from build123d import *

# Parameters (mm, degrees)
BOSS_EXTRUDE3_DEPTH = 9.25
SKETCH5_W           = 4
SKETCH5_H           = 0.86
CUT_EXTRUDE1_DEPTH  = 2
SKETCH6_W           = 3.5
SKETCH6_H           = 0.5
BOSS_EXTRUDE4_DEPTH = 0.5
SKETCH7_W           = 0.72
SKETCH7_H           = 2.3359
CUT_EXTRUDE2_DEPTH  = 2
FILLET1_R           = 0.25
FILLET2_R           = 0.1


with BuildPart() as part:
    # Sketch1 → Boss-Extrude3 (new body, symmetric)
    with BuildSketch(Plane(origin=(0, 0, 0), x_dir=(0, 0, -1), z_dir=(1, 0, 0))):
        Polygon((-0.122813016, -2.026219673), (-0.122813016, 0.173780327), (1.877186984, 0.309680327), (1.877186984, -2.026219673), align=None)
    extrude(amount=BOSS_EXTRUDE3_DEPTH, both=True)

    # Sketch5 → Cut-Extrude1 (cut)
    with BuildSketch(Plane(origin=(0, 0, -1.877186984), x_dir=(-1, 0, 0), z_dir=(0, 0, -1))):
        with Locations((-2.34, -0.120319673)):
            Rectangle(SKETCH5_W, SKETCH5_H)
    extrude(amount=-CUT_EXTRUDE1_DEPTH, mode=Mode.SUBTRACT)

    # Sketch6 → Boss-Extrude4 (add)
    with BuildSketch(Plane.XZ.offset(2.026219673)):
        with Locations((0.34, -0.877186984)):
            Rectangle(SKETCH6_W, SKETCH6_H)
    extrude(amount=BOSS_EXTRUDE4_DEPTH)

    # Sketch7 → Cut-Extrude2 (cut)
    with BuildSketch(Plane(origin=(0, 0, -1.877186984), x_dir=(-1, 0, 0), z_dir=(0, 0, -1))):
        with Locations((8.89, -0.858269673)):
            Rectangle(SKETCH7_W, SKETCH7_H)
    extrude(amount=-CUT_EXTRUDE2_DEPTH, mode=Mode.SUBTRACT)

    # Fillet1
    fillet1_edges = [part.edges().sort_by_distance(p)[0] for p in [
        (9.25, -0.858269673, -1.877186984),
        (9.25, -2.026219673, -0.877186984),
        (9.25, -0.926219673, 0.122813016),
        (-8.53, 0.241730327, -0.877186984),
        (-8.53, -0.926219673, 0.122813016),
        (-8.53, -2.026219673, -0.877186984),
        (-8.53, -0.858269673, -1.877186984),
        (9.25, 0.241730327, -0.877186984),
    ]]
    fillet(fillet1_edges, radius=FILLET1_R)

    # Fillet2
    fillet2_edges = [part.edges().sort_by_distance(p)[0] for p in [
        (-1.41, -2.526219673, -0.877186984),
        (2.09, -2.526219673, -0.877186984),
    ]]
    fillet(fillet2_edges, radius=FILLET2_R)


solid = part.part
The model under review builds one solid part; all positions refer to its coordinate system, in mm. A direction names the side the tool comes from. Round coordinates to 2 decimals unless told otherwise and drop trailing zeros. Order: outer loops, then holes, each group sorted by start corner. A loop starts at its lowest first (then second) coordinate and runs counter-clockwise, first axis right, second up. Notation, with made-up numbers: (20.5, -19) -> (54.5, -19) arc R10 cw to (54.5, -4) -> close; hole circle Ø7 at (5, 35.5). An arc over 180 degrees is marked (long way). Return JSON: item names as keys, results as strings.
1. Take a section at D-D (x = -3.5). Write out the cut boundary in (y, z), then the cut area to 3 significant figures.
Answer block:
{"outline": "(-2.03, -1.88) -> (0.31, -1.88) -> (0.17, 0.12) -> (-2.03, 0.12) -> close", "area": "4.54 mm²"}
2. Take a section at B-B (x = 1.5). Write out the cut boundary in (y, z).
Answer block:
{"outline": "(-2.53, -1.13) -> (-2.03, -1.13) -> (-2.03, -1.88) -> (-0.55, -1.88) -> (-0.55, 0.12) -> (-2.03, 0.12) -> (-2.03, -0.63) -> (-2.53, -0.63) -> close"}
3. The part is to be moulded in two halves that separate along X. For faces 3 (the face through (4.34, 0, -1)), 4 (the face through (-3.91, 0.24, -0.86)), 5 (the face through (2, -0.55, -1)), 6 (the face through (9.25, -1, -1)), say which applies: +X half, -X half, draft (parallel to the pull), parting line (faces both ways), or undercut.
Answer block:
{"face 3": "undercut", "face 4": "draft", "face 5": "undercut", "face 6": "+X half"}
4. For L1, parallel to X at y = -0.3, z = -1.3; L2, parallel to Y at x = 2, z = -0.1; L3, parallel to Z at x = 1.25, y = -2.25, list the stretches that pass through material, from the lowest coordinate up. Write a range as [from, to].
Answer block:
{"L1": "x = [-8.53, 0.34], [4.34, 9.25]", "L2": "y = [-2.03, -0.55]", "L3": "z = [-1.13, -0.63]"}
5. Insertion check: P1, Ø0.6, axis at x = 2, z = -1, coming from the +Y side; P2, Ø0.6, axis at x = -2.5, z = -0.5, coming from the -Y side; P3, Ø0.6, axis at x = 0, y = -2.5, coming from the -Z side. Each pin has a flat end and moves straight along its axis. Give the tip position at first contact, or say it passes through.
Answer block:
{"P1": "stops at y = -0.55", "P2": "stops at y = -2.03", "P3": "stops at z = -1.13"}
6. Take a section at C-C (x = -0.5). Write out the cut boundary in (y, z).
Answer block:
{"outline": "(-2.53, -1.13) -> (-2.03, -1.13) -> (-2.03, -1.88) -> (0.31, -1.88) -> (0.17, 0.12) -> (-2.03, 0.12) -> (-2.03, -0.63) -> (-2.53, -0.63) -> close"}
7. Take a section at A-A (y = -0.35). Write out the cut boundary in (x, z), then the cut area to 3 significant figures.
Answer block:
{"outline": "(-8.53, -1.63) arc R0.25 ccw to (-8.28, -1.88) -> (0.34, -1.88) -> (0.34, 0.12) -> (-8.28, 0.12) arc R0.25 ccw to (-8.53, -0.13) -> close; (4.34, -1.88) -> (9, -1.88) arc R0.25 ccw to (9.25, -1.63) -> (9.25, -0.13) arc R0.25 ccw to (9, 0.12) -> (4.34, 0.12) -> close", "area": "27.5 mm²"}
8. For faces 1 (the face through (0, -1, -1.877)), 2 (the face through (0.34, 0, -1)), list the 3-axis set-ups (+Z, -Z, +X, -X, +Y, -Y) from which the entire face can be reached by the end or side of a thin tool; tool diameter is ignored.
Answer block:
{"face 1": "-Z, +X, -X, +Y, -Y", "face 2": "+Z, -Z, +Y"}
